Geometry: final body of the model. Coordinates: model frame, mm. A direction names the side the tool comes from. Give positions to 0.01 mm unless a question says otherwise; leave off trailing zeros. Write each loop counter-clockwise with the first axis right and the second up, starting at its lowest first coordinate (ties: lowest second). Pieces come first, ordered by that corner, then holes. Notation, with made-up numbers: (-22.75, 12.25) -> (9.25, 12.25) arc R19 ccw to (9.25, 37.25) -> close; hole circle Ø10 at (60.5, -37). An arc over 180 degrees is marked (long way). Use CSV: the item, a comma, the result in double quotes. Start each with the question number.
1) Section A-A (z = 38.5). Output: boundary loops of the cut face in (x, y), plus the area to 3 significant figures.
2) Contact query for flat-ended pins moving along their axis: P1, Ø4, axis at y = 12, z = 31, coming from the +X side; P2, Ø3, axis at x = -14.5, y = -19.5, coming from the +Z side; P3, Ø2, axis at x = 4, z = -3.5, coming from the +Y side. Output: stop coordinate, or through.
3) Set-up query: faces 5 (the face through (21.35, -11.25, -5.4)), 6 (the face through (-4.47, 11.25, -14.27)), 7 (the face through (2.942, -3, -18)), 8 (the face through (-4.39, -11.17, -5.56)). Return all of +Z, -Z, +X, -X, +Y, -Y with unobstructed straight access to the full face (end or side cutting, diameter ignored); none if empty.
4) Material intervals for line 1 (Z direction, x = 17, y = -20); line 2 (Y direction, x = -1.5, z = 3); line 3 (Z direction, x = 4.5, y = -15), sorted ascending. Write a range as [from, to].
5) Section B-B (z = 14). Output: boundary loops of the cut face in (x, y).
6) Draft query along Y for faces 1 (the face through (23.208, -23.616, 30.989)), 2 (the face through (24.78, -4.33, 21.83)), 3 (the face through (-23.862, -4.327, 27.464)), 4 (the face through (-24.671, -2.127, 22.756)). Return one class per face: pulls with the +Y half, pulls with the -Y half, needs draft (parallel to the pull), parting line crosses it, or undercut.
```python
from build123d import *

# Parameters (mm, degrees)
F0_W      = 19.9313152116
F0_H      = 28.9478618652
F1_DEPTH  = 12.7
F2_W      = 19.9313152116
F2_H      = 12.9078961909
F3_DEPTH  = 12.7
F4_F1_R   = 5.08
F4_F2_R   = 5.08
F8_DEPTH  = 6.2511
F10_DEPTH = 6.35


with BuildPart() as f1:
    # F0 (on Front) → F1 (new body, symmetric)
    with BuildSketch(Plane.XZ):
        Polygon((22.873558104, 0), (25.4, 0), (18.9548347086, 37.5508967185), (0, 37.5508967185), (0, 0), (2.9422428925, 0), align=None)
        with Locations((12.9079004982, -14.4739309326)):
            Rectangle(F0_W, F0_H)
        Polygon((0, 0), (0, 37.5508967185), (-18.9548347086, 37.5508967185), (-25.4, 0), (-22.873558104, 0), (-2.9422428925, 0), align=None)
        with Locations((-12.9079004982, -14.4739309326)):
            Rectangle(F0_W, F0_H)
    extrude(amount=F1_DEPTH, both=True)

    # F2 (on face) → F3 (join)
    with BuildSketch(Plane.XZ.offset(12.7)):
        with Locations((12.9079004982, -22.4939137697)):
            Rectangle(F2_W, F2_H)
        with Locations((-12.9079004982, -22.4939137697)):
            Rectangle(F2_W, F2_H)
    extrude(amount=F3_DEPTH)

    # F4: fillet of radius 5.08 on 18 edges, made by hand

    # F4_f1
    f4_f1_edges = [f1.edges().sort_by_distance(p)[0] for p in [
        (12.9079004982, -12.7, -16.0399656743),
        (-12.9079004982, -12.7, -16.0399656743),
    ]]
    fillet(f4_f1_edges, radius=F4_F1_R)

    # F4_f2
    f4_f2_edges = [f1.edges().sort_by_distance(p)[0] for p in [
        (-2.9422428925, -25.4, -22.4939137697),
        (-12.9079004982, -25.4, -16.0399656743),
        (-22.873558104, -25.4, -22.4939137697),
        (-12.9079004982, -25.4, -28.9478618652),
        (22.873558104, -25.4, -22.4939137697),
        (12.9079004982, -25.4, -16.0399656743),
        (2.9422428925, -25.4, -22.4939137697),
        (12.9079004982, -25.4, -28.9478618652),
        (-2.9422428925, -21.59, -16.0399656743),
        (-22.873558104, -21.59, -16.0399656743),
        (22.873558104, 12.7, -14.4739309326),
        (2.9422428925, 12.7, -14.4739309326),
        (-22.873558104, 12.7, -14.4739309326),
        (-2.9422428925, 12.7, -14.4739309326),
        (22.873558104, -12.7, -5.4799828371),
        (2.9422428925, -12.7, -5.4799828371),
        (2.9422428925, -14.1878975516, -14.5520681227),
        (22.873558104, -14.1878975516, -14.5520681227),
        (-22.873558104, -14.1878975516, -14.5520681227),
        (-2.9422428925, -14.1878975516, -14.5520681227),
    ]]
    fillet(f4_f2_edges, radius=F4_F2_R)

    # F5 (on Front) → F6 (revolve)
    with BuildSketch(Plane.XZ):
        with BuildLine():
            Line((7.6877931133, 33.1239514053), (7.6877931133, 40.7419648703))
            ThreePointArc((7.6877931133, 40.7419648703), (16.6857685514, 50.0178025185), (7.8776162118, 59.4740797153))
            Line((7.8776162118, 59.4740797153), (7.8776162118, 61.787083745))
            Line((7.8776162118, 61.787083745), (0, 61.787083745))
            Line((0, 61.787083745), (0, 33.1239514053))
            Line((0, 33.1239514053), (7.6877931133, 33.1239514053))
        make_face()
    revolve(axis=Axis((0, 0, 47.4555175751), (0, 0, 1)))

    # F7 (on face) → F8 (join)
    with BuildSketch(Plane(origin=(24.6731381341, 0, 4.234851027), x_dir=(0, 1, 0), z_dir=(0.9855878404, 0, 0.1691644433))):
        with BuildLine():
            Line((-12.7, 16.9602958167), (4.2709973641, 17.6954660565))
            ThreePointArc((4.2709973641, 17.6954660565), (11.5417566939, 23.7592524776), (3.2686796257, 28.3624733953))
            Line((3.2686796257, 28.3624733953), (-9.0165464208, 22.251194343))
            Line((-9.0165464208, 22.251194343), (-22.1028998209, 29.3900118281))
            Line((-22.1028998209, 29.3900118281), (-25.1719959147, 23.7639713547))
            Line((-25.1719959147, 23.7639713547), (-12.7, 16.9602958167))
        make_face()
    extrude(amount=F8_DEPTH)

    # F9 (on face) → F10 (join)
    with BuildSketch(Plane(origin=(-24.6731381341, 0, 4.234851027), x_dir=(0, -1, 0), z_dir=(-0.9855878404, 0, 0.1691644433))):
        with BuildLine():
            Line((10.2126034461, 20.4402103872), (-1.7259411979, 25.6970115006))
            ThreePointArc((-1.7259411979, 25.6970115006), (-8.7725675478, 30.2032799266), (-6.2509044074, 22.2281552851))
            Line((-6.2509044074, 22.2281552851), (10.7428459451, 14.1681702808))
            Line((10.7428459451, 14.1681702808), (12.7, 15.2765091522))
            Line((12.7, 15.2765091522), (12.7, 21.8488262713))
            Line((12.7, 21.8488262713), (10.2126034461, 20.4402103872))
        make_face()
        Polygon((20.8962647478, 26.4903815939), (12.7, 21.8488262713), (12.7, 15.2765091522), (23.7144064158, 21.5139817446), align=None)
    extrude(amount=F10_DEPTH)


solid = f1.part
```
Answers follow:
1,outline,"circle Ø15.38 at (0, 0)"
1,area,"186 mm^2"
2,P1,"stops at x = 26.75"
2,P2,"stops at z = -16.04"
2,P3,"stops at y = 11.7"
3,face 5,"+X, -Y"
3,face 6,"-Z, +Y"
3,face 7,"-Z, +Y, -Y"
3,face 8,"-Y"
4,line 1,"z = [-28.95, -16.04]"
4,line 2,"y = [-12.7, 12.7]"
4,line 3,"z = [-28.95, -16.83], [45.85, 54.38]"
5,outline,"(-23, -12.7) -> (23, -12.7) -> (23, 12.7) -> (-23, 12.7) -> close"
6,face 1,"pulls with the -Y half"
6,face 2,"undercut"
6,face 3,"undercut"
6,face 4,"pulls with the +Y half"
